Geometry: final body of the model. Coordinates: model frame, mm. Face numbers are marked on the shaded views. A direction names the side the tool comes from. Give positions to 0.01 mm unless a question says otherwise; leave off trailing zeros. Write each loop counter-clockwise with the first axis right and the second up, starting at its lowest first coordinate (ties: lowest second). Pieces come first, ordered by that corner, then holes. Notation, with made-up numbers: M 71.5,9 L 82.5,9 A27 ccw 82.5,37 Z; hole C 46.25,-40 d2. An arc over 180 degrees is marked long. One line per question, with ' | ' between items.
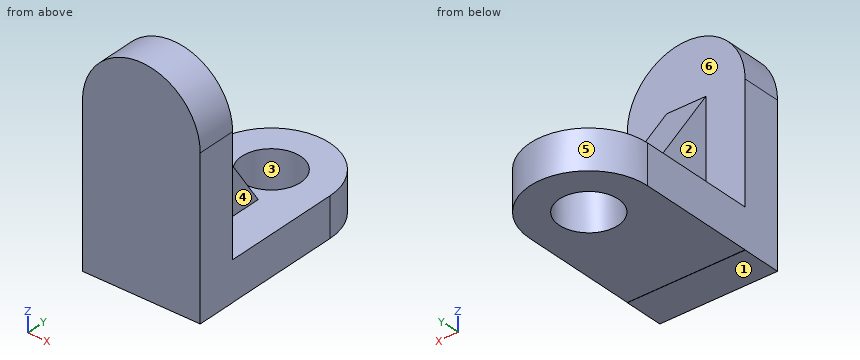
Solid Edge part; units mm, degrees
sketch "Sketch1" plane through (0, 0, 0) normal (0, 0, 1) x (1, 0, 0)
  line L0 (15, 0) -> (15, 40)
  line L1 (-15, 0) -> (15, 0)
  line L2 (-15, 40) -> (-15, 0)
  arc A0 (-15, 40) -> (15, 40) centre (0, 40) cw
extrude "Protrusion1" add sketch "Sketch1" against normal blind 10
sketch "Sketch2" plane through (0, 0, 0) normal (0, 0, 1) x (1, 0, 0)
  circle A0 centre (0, 40) radius 7.5
extrude "ExtrudedCutout_2" cut sketch "Sketch2" against normal blind 10
sketch "Sketch3" plane through (-15, 20, -5) normal (-1, 0, 0) x (0, 0, 1)
  line L0 (34.9554, -10.0744) -> (-5.0446, -10.0744)
  line L1 (-5.0446, -10.0744) -> (-5.0446, -20.0744)
  line L2 (-5.0446, -20.0744) -> (34.9554, -20.0744)
  line L3 (34.9554, -20.0744) -> (34.9554, -10.0744)
extrude "ExtrudedProtrusion_2" add sketch "Sketch3" against normal blind 30
sketch "Sketch4" plane through (0, 9.9256, 14.9777) normal (0, 1, 0) x (1, 0, 0)
  arc A0 (14.9999, -14.9131) -> (-14.9999, -14.9131) centre (0, -14.9777) cw
extrude "ExtrudedProtrusion_3" add sketch "Sketch4" against normal blind 10 material side at (0, 9.9256, 44.9054)
sketch "Sketch5" plane through (0, 0, 0) normal (1, 0, 0) x (0, 1, 0)
  line L0 (9.9256, 30) -> (29.9256, 0)
  line L1 (9.9256, 0) -> (29.9256, 0)
  line L2 (9.9256, 0) -> (9.9256, 30)
extrude "ExtrudedProtrusion_5" add sketch "Sketch5" along normal blind 5
sketch "Sketch6" plane through (0, 0, 0) normal (1, 0, 0) x (0, 1, 0)
  line L0 (9.9256, 30) -> (29.9256, 0)
  line L1 (9.9256, 0) -> (29.9256, 0)
  line L2 (9.9256, 0) -> (9.9256, 30)
extrude "ExtrudedProtrusion_6" add sketch "Sketch6" against normal blind 5
(1) Cut plane C-C, the plane y = 22.5. Return loops of the section in (x, z), then the cut area to 3 significant figures.
Working result:
outline: M -15,-10 L 15,-10 L 15,0 L 5,0 L 5,11.14 L -5,11.14 L -5,0 L -15,0 Z | area: 411 mm^2
(2) Cut plane D-D, the plane z = 35.5. Return loops of the section in (x, y).
Working result:
outline: M -13.94,-0.07 L 13.94,-0.07 L 13.94,9.93 L -13.94,9.93 Z
(3) Material intervals for L1, parallel to Y at x = 0, z = -5; L2, parallel to Y at x = -11.25, z = 9; L3, parallel to Z at x = -10.5, y = 10, sorted ascending. Write a range as [from, to].
Working result:
L1: y = [-0.07, 32.5], [47.5, 55] | L2: y = [-0.07, 9.93] | L3: z = [-10, 0]
(4) Cut plane A-A, the plane x = 0. Return loops of the section in (y, z), then the cut area to 3 significant figures.
Working result:
outline: M -0.07,-10.04 L 9.93,-10.04 L 9.93,-10 L 32.5,-10 L 32.5,0 L 29.93,0 L 9.93,30 L 9.93,44.96 L -0.07,44.96 Z; M 47.5,-10 L 55,-10 L 55,0 L 47.5,0 Z | area: 1,150 mm^2
(5) Draft query along X for the marked faces 1, 2 and 3. Return one class per face: released by +X, released by -X, zero draft, split by the parting line, or undercut.
Working result:
face 1: zero draft | face 2: released by -X | face 3: undercut
(6) First-contact query: P1, Ø1, axis at x = -5.5, y = 48, coming from the +Z side; P2, Ø15, axis at x = 6.5, y = 35, coming from the -Z side; P3, Ø16, axis at y = 18.5, z = 20.5, coming from the +X side. Flat tips, straight axial feed; report the tip coordinate or a pass-through.
Working result:
P1: stops at z = 0 | P2: stops at z = -10 | P3: stops at x = 5
(7) Cut plane B-B, the plane x = -8.25. Return loops of the section in (y, z).
Working result:
outline: M -0.07,-10.04 L 9.93,-10.04 L 9.93,-10 L 52.53,-10 L 52.53,0 L 9.93,0 L 9.93,42.48 L -0.07,42.48 Z
(8) Set-up query: the marked faces 4, 5 and 6. Return all of +Z, -Z, +X, -X, +Y, -Y with unobstructed straight access to the full face (end or side cutting, diameter ignored); none if empty.
Working result:
face 4: +Z, +X, +Y | face 5: +Z, -Z, +Y | face 6: +Z, +Y
